CAD build for the part. Positions are in the model's coordinates, mm. A direction names the side the tool comes from. Round coordinates to 2 decimals unless told otherwise and drop trailing zeros. Write each loop counter-clockwise with the first axis right and the second up, starting at its lowest first coordinate (ties: lowest second). Pieces come first, ordered by that corner, then holes. Notation, with made-up numbers: (43.25, -18) - (74.25, -18) arc R32 cw to (74.25, 17) - close; hole circle Ø4 at (53.5, 27.25). An arc over 180 degrees is marked (long way). Put each result on its own line as item: value. Start each with the question number.
Item 1: Mould opens along Y. For faces 1 (the flat face through (-15, 15, -551)), 2 (the flat face through (0, 28, -551)), 3 (the flat face through (0, 30, -551)), 4 (the flat face through (0, 0, -551)) say: released by +Y, released by -Y, zero draft, split by the parting line, or undercut.
Item 2: Cut at B-B (x = -2). Give the cut face in (y, z).
Item 3: Cut at A-A (y = 11.75). Give the cut face in (x, z).
Item 4: Cut at C-C (z = -594). Give the cut face in (x, y).
Item 5: 3-axis set-ups, long thin cutter, end or side, ignore diameter. For faces 5 (the flat face through (0, 2, -551)), 6 (the flat face through (0, 29, -1078)): which of +Z, -Z, +X, -X, +Y, -Y reach the whole face in a straight line?
Item 6: Drill centre lines: line 1 (Y direction, x = -11, z = -188.5); line 2 (X direction, y = 18.75, z = -206); line 3 (Y direction, x = -12.5, z = -639.5). Where is each one in solid material? Low to high. Write a range as from..to.
```python
from build123d import *

# Parameters (mm, degrees)
EXTRUDE_1_DEPTH = 534


with BuildPart() as part:
    # Эскиз1 → Бобышка-Вытянуть1 (new body)
    with BuildSketch(Plane.XY.offset(-10)):
        with BuildLine():
            Line((12, 0), (-12, 0))
            ThreePointArc((-12, 0), (-14.121320344, 0.878679656), (-15, 3))
            Line((-15, 3), (-15, 27))
            ThreePointArc((-15, 27), (-14.121320344, 29.121320344), (-12, 30))
            Line((-12, 30), (12, 30))
            ThreePointArc((12, 30), (14.121320344, 29.121320344), (15, 27))
            Line((15, 27), (15, 3))
            ThreePointArc((15, 3), (14.121320344, 0.878679656), (12, 0))
        make_face()
        with BuildLine():
            Line((11, 2), (-11, 2))
            ThreePointArc((-11, 2), (-12.414213562, 2.585786438), (-13, 4))
            Line((-13, 4), (-13, 26))
            ThreePointArc((-13, 26), (-12.414213562, 27.414213562), (-11, 28))
            Line((-11, 28), (11, 28))
            ThreePointArc((11, 28), (12.414213562, 27.414213562), (13, 26))
            Line((13, 26), (13, 4))
            ThreePointArc((13, 4), (12.414213562, 2.585786438), (11, 2))
        make_face(mode=Mode.SUBTRACT)
    extrude(amount=-EXTRUDE_1_DEPTH)

    # Зеркальное отражение1: part across plane


with BuildPart() as part_1:
    add(part.part)
    add(part.part.mirror(Plane(origin=(695.566765073, 158.190477347, -544), x_dir=(1, 0, 0), z_dir=(0, 0, 1))))


solid = part_1.part
```
Output values:
1. face 1: zero draft
1. face 2: undercut
1. face 3: released by +Y
1. face 4: released by -Y
2. outline: (0, -1078) - (2, -1078) - (2, -10) - (0, -10) - close; (28, -1078) - (30, -1078) - (30, -10) - (28, -10) - close
3. outline: (-15, -1078) - (-13, -1078) - (-13, -10) - (-15, -10) - close; (13, -1078) - (15, -1078) - (15, -10) - (13, -10) - close
4. outline: (-15, 3) arc R3 ccw to (-12, 0) - (12, 0) arc R3 ccw to (15, 3) - (15, 27) arc R3 ccw to (12, 30) - (-12, 30) arc R3 ccw to (-15, 27) - close; hole (-13, 4) arc R2 ccw to (-11, 2) - (11, 2) arc R2 ccw to (13, 4) - (13, 26) arc R2 ccw to (11, 28) - (-11, 28) arc R2 ccw to (-13, 26) - close
5. face 5: +Z, -Z
5. face 6: -Z, +X, -X, +Y, -Y
6. line 1: 0..2, 28..30
6. line 2: -15..-13, 13..15
6. line 3: 0.04..2.68, 27.32..29.96
